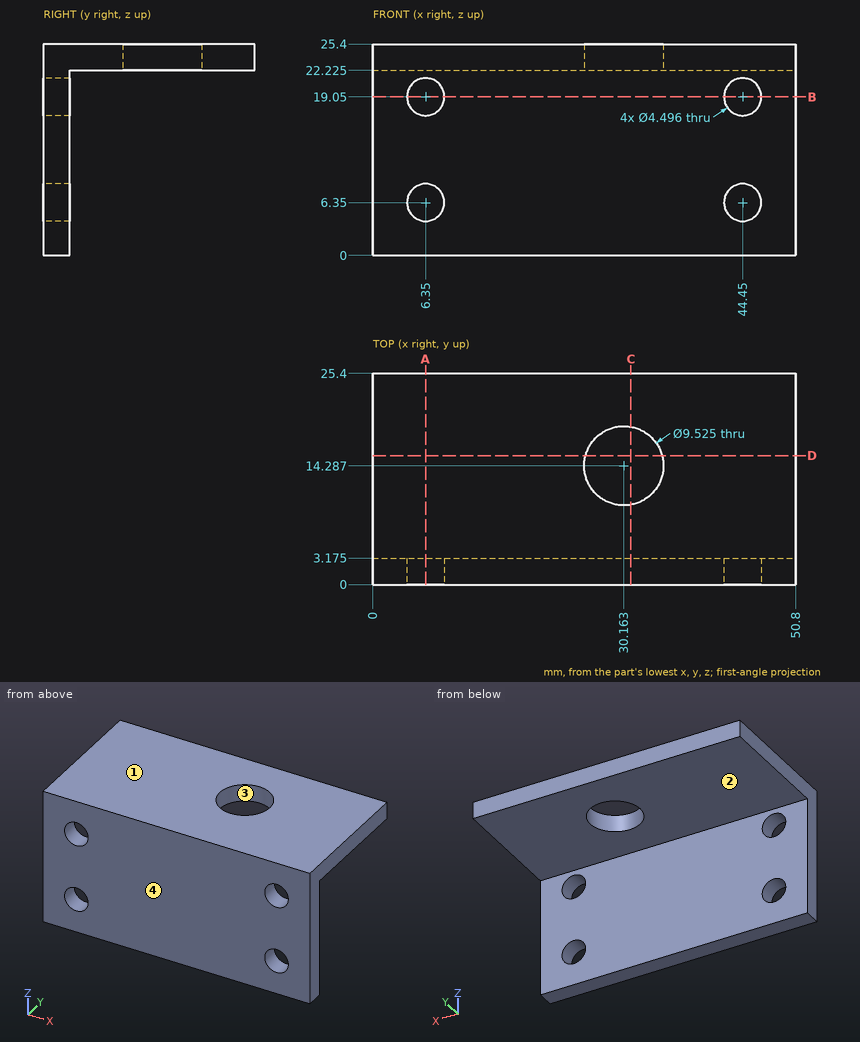
Design review of the part shown in the three views and the two pictorial views. Dimensions are in mm from the part's minimum x, y and z. A direction names the side the tool comes from. Round coordinates to 2 decimals unless told otherwise and drop trailing zeros. Write each loop counter-clockwise with the first axis right and the second up, starting at its lowest first coordinate (ties: lowest second). Pieces come first, ordered by that corner, then holes.
Item 1: We need section B-B on z = 19.05. Write out the cut boundary in (x, y) (1 decimal), and give its area (3 significant figures).
Item 2: The part is to be moulded in two halves that separate along X. For the marked faces 3 and 4, say which applies: +X half, -X half, draft (parallel to the pull), parting line (faces both ways), or undercut.
Item 3: We need section D-D on y = 15.5. Write out the cut boundary in (x, z) (1 decimal), and give its area (3 significant figures).
Item 4: Clearance check with flat-ended pins moving along their axes: pin 1 Ø4 at (x, y) = (26, 17) entering from -Z (1 decimal); pin 2 Ø2.5 at (x, z) = (6.35, 19.05) entering from -Y; pin 3 Ø6 at (x, z) = (44.45, 6.35) entering from +Y (1 decimal). State where each tip first meets the part, or that it passes through.
Item 5: We need section C-C on x = 31. Write out the cut boundary in (y, z) (1 decimal).
Item 6: For the marked faces 1 and 2, list the 3-axis set-ups (+Z, -Z, +X, -X, +Y, -Y) from which the entire face can be reached by the end or side of a thin tool; tool diameter is ignored.
Item 7: For probe 1 along Z at (x, y) = (44.45, 1.2); probe 2 along Z at (x, y) = (39, 21.25) (1 decimal); probe 3 along Y at (x, z) = (10, 5) (1 decimal), list the stretches that pass through material, from the lowest coordinate up.
Item 8: We need section A-A on x = 6.35. Write out the cut boundary in (y, z) (1 decimal).
Returned:
1. outline: (0, 0) - (4.1, 0) - (4.1, 3.2) - (0, 3.2) - close; (8.6, 0) - (42.2, 0) - (42.2, 3.2) - (8.6, 3.2) - close; (46.7, 0) - (50.8, 0) - (50.8, 3.2) - (46.7, 3.2) - close
1. area: 133 mm2
2. face 3: undercut
2. face 4: draft
3. outline: (0, 22.2) - (25.6, 22.2) - (25.6, 25.4) - (0, 25.4) - close; (34.8, 22.2) - (50.8, 22.2) - (50.8, 25.4) - (34.8, 25.4) - close
3. area: 132 mm2
4. pin 1: stops at z = 22.2
4. pin 2: passes through
4. pin 3: stops at y = 3.2
5. outline: (0, 0) - (3.2, 0) - (3.2, 22.2) - (9.6, 22.2) - (9.6, 25.4) - (0, 25.4) - close; (19, 22.2) - (25.4, 22.2) - (25.4, 25.4) - (19, 25.4) - close
6. face 1: +Z, +X, -X, +Y, -Y
6. face 2: -Z, +X, -X, +Y
7. probe 1: z = 0 to 4.1, 8.6 to 16.8, 21.3 to 25.4
7. probe 2: z = 22.2 to 25.4
7. probe 3: y = 0 to 3.2
8. outline: (0, 0) - (3.2, 0) - (3.2, 4.1) - (0, 4.1) - close; (0, 8.6) - (3.2, 8.6) - (3.2, 16.8) - (0, 16.8) - close; (0, 21.3) - (3.2, 21.3) - (3.2, 22.2) - (25.4, 22.2) - (25.4, 25.4) - (0, 25.4) - close
